Part model, mm, in its own coordinate system. Face numbers are marked on the shaded views. Round coordinates to 2 decimals unless told otherwise and drop trailing zeros. Write each loop counter-clockwise with the first axis right and the second up, starting at its lowest first coordinate (ties: lowest second). Pieces come first, ordered by that corner, then holes.
```python
from build123d import *

# Parameters (mm, degrees)
SKETCH_2_W                = 45
SKETCH_2_H                = 33
SKETCH_2_R                = 1.5
EXTRUDE_1_DEPTH           = 6
SKETCH_3_W                = 45
SKETCH_3_H                = 3
EXTRUDE_2_DEPTH           = 2
SKETCH_4_R                = 3.5
CUT_EXTRUDE_1_DEPTH       = 2
SKETCH_11_W               = 45
SKETCH_11_H               = 3
EXTRUDE_4_DEPTH           = 8
CUT_EXTRUDE_2_REACH       = 10
SKETCH_9_W                = 12.05
SKETCH_9_H                = 3
CHAMFER_1_SIZE            = 0.5
SKETCH_19_W               = 6
SKETCH_19_H               = 6
CUT_EXTRUDE_4_DEPTH       = 2
HOLE_WIZARD_3_0_3_1_D     = 3
HOLE_WIZARD_3_0_3_1_DEPTH = 6.001
CHAMFER_2_SIZE            = 0.5
SKETCH_20_W               = 15
SKETCH_20_H               = 26
CUT_EXTRUDE_5_DEPTH       = 2
FILLET_1_R                = 1
SKETCH_22_W               = 15
SKETCH_22_H               = 6
CUT_EXTRUDE_6_DEPTH       = 2


with BuildPart() as part:
    # 草图2 → 凸台-拉伸1 (new body)
    with BuildSketch(Plane(origin=(0, 0, 0), x_dir=(1, 0, 0), z_dir=(0, 1, 0))):
        Rectangle(SKETCH_2_W, SKETCH_2_H)
        with Locations((-7.5, 10)):
            Circle(SKETCH_2_R, mode=Mode.SUBTRACT)
        with Locations((7.5, 10)):
            Circle(SKETCH_2_R, mode=Mode.SUBTRACT)
        with Locations((-7.5, -10)):
            Circle(SKETCH_2_R, mode=Mode.SUBTRACT)
        with Locations((7.5, -10)):
            Circle(SKETCH_2_R, mode=Mode.SUBTRACT)
    extrude(amount=EXTRUDE_1_DEPTH)

    # 草图3 → 凸台-拉伸2 (add)
    with BuildSketch(Plane.XZ):
        with Locations((0, -15)):
            Rectangle(SKETCH_3_W, SKETCH_3_H)
        with Locations((0, 15)):
            Rectangle(SKETCH_3_W, SKETCH_3_H)
    extrude(amount=EXTRUDE_2_DEPTH)

    # 草图4 → 切除-拉伸1 (cut)
    with BuildSketch(Plane(origin=(0, 6, 0), x_dir=(1, 0, 0), z_dir=(0, 1, 0))):
        with Locations((-7.5, 10)):
            Circle(SKETCH_4_R)
        with Locations((7.5, 10)):
            Circle(SKETCH_4_R)
        with Locations((7.5, -10)):
            Circle(SKETCH_4_R)
        with Locations((-7.5, -10)):
            Circle(SKETCH_4_R)
    extrude(amount=-CUT_EXTRUDE_1_DEPTH, mode=Mode.SUBTRACT)

    # 草图11 → 凸台-拉伸4 (add)
    with BuildSketch(Plane(origin=(0, 6, 0), x_dir=(1, 0, 0), z_dir=(0, 1, 0))):
        with Locations((0, 18)):
            Rectangle(SKETCH_11_W, SKETCH_11_H)
        with Locations((0, -18)):
            Rectangle(SKETCH_11_W, SKETCH_11_H)
    extrude(amount=-EXTRUDE_4_DEPTH)

    # 草图9 → 切除-拉伸2 (cut, up to next)
    with BuildSketch(Plane(origin=(0, 6, 0), x_dir=(1, 0, 0), z_dir=(0, 1, 0)), mode=Mode.PRIVATE) as cut_extrude_2_sk1:
        with Locations((0, 18)):
            Rectangle(SKETCH_9_W, SKETCH_9_H)
    cut_extrude_2_tool1 = extrude(cut_extrude_2_sk1.sketch, amount=-CUT_EXTRUDE_2_REACH, mode=Mode.PRIVATE) & part.part
    add(cut_extrude_2_tool1.solids().sort_by_distance((0, 6, -18))[0], mode=Mode.SUBTRACT)
    # 草图9 → 切除-拉伸2 (cut, up to next)
    with BuildSketch(Plane(origin=(0, 6, 0), x_dir=(1, 0, 0), z_dir=(0, 1, 0)), mode=Mode.PRIVATE) as cut_extrude_2_sk2:
        with Locations((0, -18)):
            Rectangle(SKETCH_9_W, SKETCH_9_H)
    cut_extrude_2_tool2 = extrude(cut_extrude_2_sk2.sketch, amount=-CUT_EXTRUDE_2_REACH, mode=Mode.PRIVATE) & part.part
    add(cut_extrude_2_tool2.solids().sort_by_distance((0, 6, 18))[0], mode=Mode.SUBTRACT)

    # 倒角1
    chamfer_1_edges = [part.edges().sort_by_distance(p)[0] for p in [
        (-6.025, 6, -18),
        (0, 6, -16.5),
        (6.025, 6, -18),
        (6.025, 6, 18),
        (0, 6, 16.5),
        (-6.025, 6, 18),
    ]]
    chamfer(chamfer_1_edges, length=CHAMFER_1_SIZE)

    # 草图15 → M3 螺纹孔2 (revolve, cut)
    with BuildSketch(Plane(origin=(-17.5, -2, -16.5), x_dir=(0, 0, -1), z_dir=(1, 0, 0))):
        Polygon((0, 0), (0, 4.690989712), (1.15, 4), (1.15, 0), align=None)
    hole_wizard_m3_2 = revolve(axis=Axis((-17.5, -8.35, -16.5), (0, 1, 0)), mode=Mode.SUBTRACT)

    # 草图17 → M3 螺纹孔3 (revolve, cut)
    with BuildSketch(Plane(origin=(17.5, -2, -16.5), x_dir=(0, 0, -1), z_dir=(1, 0, 0))):
        Polygon((0, 0), (0, 4.690989712), (1.15, 4), (1.15, 0), align=None)
    hole_wizard_m3_3 = revolve(axis=Axis((17.5, -8.35, -16.5), (0, 1, 0)), mode=Mode.SUBTRACT)

    # 草图19 → 切除-拉伸4 (cut)
    with BuildSketch(Plane.XZ.offset(2)):
        with Locations((-10.5, -16.5)):
            Rectangle(SKETCH_19_W, SKETCH_19_H)
        with Locations((10.5, -16.5)):
            Rectangle(SKETCH_19_W, SKETCH_19_H)
    cut_extrude_4 = extrude(amount=-CUT_EXTRUDE_4_DEPTH, mode=Mode.SUBTRACT)

    # Ø3.0 (3) 直径孔1
    with Locations(Plane.XZ):
        with Locations((-10.5, -16.5), (10.5, -16.5)):
            hole_wizard_3_0_3_1 = Hole(HOLE_WIZARD_3_0_3_1_D / 2, depth=HOLE_WIZARD_3_0_3_1_DEPTH)

    # 镜向1: M3 螺纹孔2, M3 螺纹孔3, 切除-拉伸4, Ø3.0 (3) 直径孔1 across plane
    add(hole_wizard_m3_2.mirror(Plane.XY), mode=Mode.SUBTRACT)
    add(hole_wizard_m3_3.mirror(Plane.XY), mode=Mode.SUBTRACT)
    add(cut_extrude_4.mirror(Plane.XY), mode=Mode.SUBTRACT)
    add(hole_wizard_3_0_3_1.mirror(Plane.XY), mode=Mode.SUBTRACT)

    # 倒角2
    chamfer_2_edges = [part.edges().sort_by_distance(p)[0] for p in [
        (-18, -2, -13.5),
        (0, -2, -13.5),
        (0, -2, 13.5),
        (18, -2, 13.5),
        (18, -2, -13.5),
        (-18, -2, 13.5),
    ]]
    chamfer(chamfer_2_edges, length=CHAMFER_2_SIZE)

    # 草图20 → 切除-拉伸5 (cut)
    with BuildSketch(Plane(origin=(0, 6, 0), x_dir=(1, 0, 0), z_dir=(0, 1, 0))):
        with Locations((15, 0)):
            Rectangle(SKETCH_20_W, SKETCH_20_H)
        with Locations((-15, 0)):
            Rectangle(SKETCH_20_W, SKETCH_20_H)
    extrude(amount=-CUT_EXTRUDE_5_DEPTH, mode=Mode.SUBTRACT)

    # 圆角1
    fillet_1_edges = [part.edges().sort_by_distance(p)[0] for p in [
        (9.302775638, 5, 13),
        (7.5, 5, 6.5),
        (7.5, 5, -6.5),
        (9.302775638, 5, -13),
        (-9.302775638, 5, -13),
        (-7.5, 5, -6.5),
        (-7.5, 5, 6.5),
        (-9.302775638, 5, 13),
    ]]
    fillet(fillet_1_edges, radius=FILLET_1_R)

    # 草图22 → 切除-拉伸6 (cut)
    with BuildSketch(Plane.XZ.offset(2)):
        with Locations((0, 16.5)):
            Rectangle(SKETCH_22_W, SKETCH_22_H)
        with Locations((0, -16.5)):
            Rectangle(SKETCH_22_W, SKETCH_22_H)
    extrude(amount=-CUT_EXTRUDE_6_DEPTH, mode=Mode.SUBTRACT)


solid = part.part
```
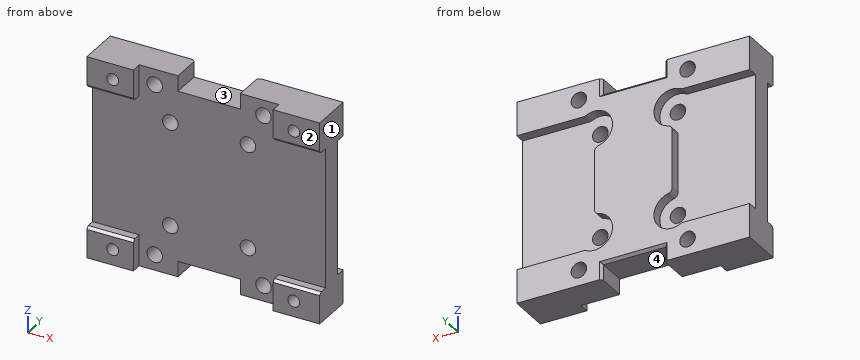
Q1. Cut at A-A on y = -0.5. Write the cut outline in (x, z).
Values follow:
outline: (-22.5, -19.5) - (-13.5, -19.5) - (-13.5, -13.5) - (-22.5, -13.5) - close; (-22.5, 13.5) - (-13.5, 13.5) - (-13.5, 19.5) - (-22.5, 19.5) - close; (13.5, -19.5) - (22.5, -19.5) - (22.5, -13.5) - (13.5, -13.5) - close; (13.5, 13.5) - (22.5, 13.5) - (22.5, 19.5) - (13.5, 19.5) - close; hole circle Ø2.3 at (-17.5, -16.5); hole circle Ø2.3 at (-17.5, 16.5); hole circle Ø2.3 at (17.5, -16.5); hole circle Ø2.3 at (17.5, 16.5)
Q2. Cut at D-D on z = 2. Write the cut outline in (x, y), plus the area to 3 significant figures.
Values follow:
outline: (-22.5, 0) - (22.5, 0) - (22.5, 4) - (7.5, 4) - (7.5, 6) - (-7.5, 6) - (-7.5, 4) - (-22.5, 4) - close
area: 210 mm2
Q3. Wall check: L1, parallel to Z at x = 10.5, y = 3.25; L2, parallel to Z at x = 17.5, y = -0.3; L3, parallel to Z at x = 7.5, y = 2.45. Give the ranges that are in metal, low to high.
Values follow:
L1: z = -19.5 to -18, -15 to 15, 18 to 19.5
L2: z = -19.5 to -17.65, -15.35 to -13.5, 13.5 to 15.35, 17.65 to 19.5
L3: z = -19.5 to -11.5, -8.5 to 8.5, 11.5 to 19.5
Q4. Cut at B-B on x = 10.5. Write the cut outline in (y, z).
Values follow:
outline: (0, -19.5) - (6, -19.5) - (6, -18) - (0, -18) - close; (0, -15) - (6, -15) - (6, -13) - (4, -13) - (4, 13) - (6, 13) - (6, 15) - (0, 15) - close; (0, 18) - (6, 18) - (6, 19.5) - (0, 19.5) - close
Q5. Cut at C-C on z = -10. Write the cut outline in (x, y).
Values follow:
outline: (-22.5, 0) - (-9, 0) - (-9, 4) - (-22.5, 4) - close; (-6, 0) - (6, 0) - (6, 4) - (4, 4) - (4, 6) - (-4, 6) - (-4, 4) - (-6, 4) - close; (9, 0) - (22.5, 0) - (22.5, 4) - (9, 4) - close
Q6. Drop flat-ended pins along their axis: pin 1 (4 mm diameter, centred on x = 7.5, z = -10, fed in from -Y); pin 2 (1.8 mm diameter, centred on x = 10.5, z = 16.5, fed in from +Y); pin 3 (1.5 mm diameter, centred on x = 13, z = 8.5, fed in from +Y); pin 4 (3 mm diameter, centred on x = -0.5, y = 1.5, fed in from +Z). Give the stop position or say it passes through.
Values follow:
pin 1: stops at y = 0
pin 2: passes through
pin 3: stops at y = 4
pin 4: stops at z = 16.5
Q7. Mould opens along X. For the marked faces 1, 2, 3 and 4 say: +X half, -X half, draft (parallel to the pull), parting line (faces both ways), or undercut.
Values follow:
face 1: +X half
face 2: draft
face 3: undercut
face 4: undercut
